For this review, use the dimensioned drawing (mm, ordinates from the lowest corner) and the shaded views. Give positions to 0.01 mm unless a question says otherwise; leave off trailing zeros. Loops run counter-clockwise (first coordinate to the right, second up) from the corner with the lowest first, then second, coordinate; pieces in that order, holes last. Notation, with made-up numbers: M 65.5,53.25 L 99.5,53.25 A11 cw 99.5,60.25 Z; hole C 10,14 d1. An arc over 180 degrees is marked long. Return JSON: item names as keys, results as strings.
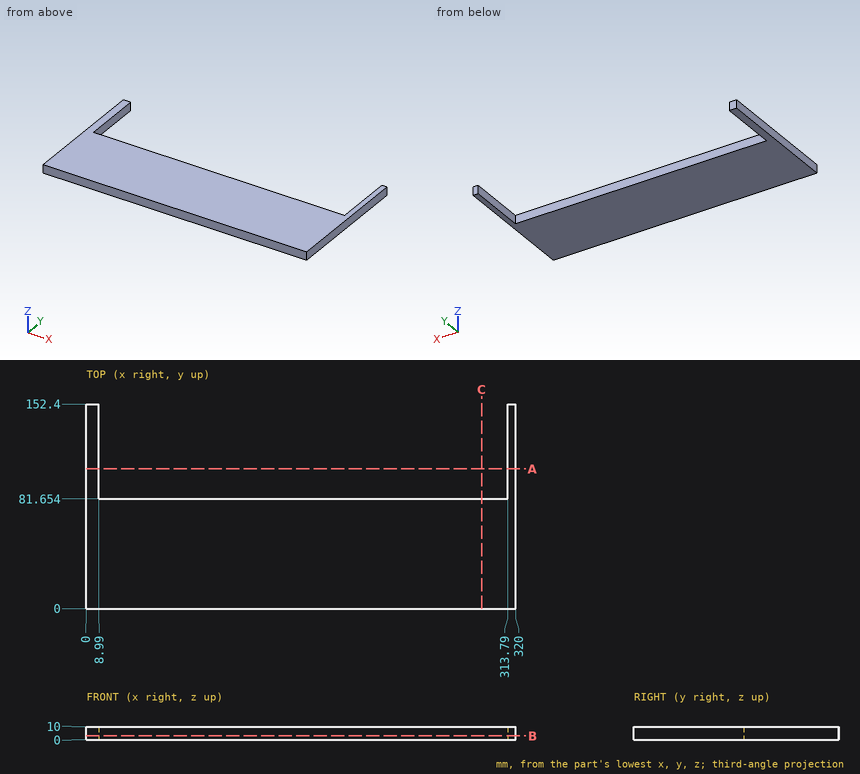
1) Insertion check: pin 1 (1 mm diameter, centred on x = 122.5, z = 5, fed in from +Y). The pin has a flat end and moves straight along its axis. Give the tip position at first contact, or say it passes through.
From the geometry:
{"pin 1": "y = 81.65"}
2) Consider section B-B on z = 3. Write out the cut boundary in (x, y), then the cut area to 3 significant figures.
From the geometry:
{"outline": "M 0,0 L 320,0 L 320,152.4 L 313.79,152.4 L 313.79,81.65 L 8.99,81.65 L 8.99,152.4 L 0,152.4 Z", "area": "27,200 mm²"}
3) Wall thickness on L1, parallel to X at y = 91, z = 5.5; L2, parallel to Y at x = 282, z = 6.75: over which ranges is each line inside the solid? List them lowest first. Write a range as from..to.
From the geometry:
{"L1": "0..8.99, 313.79..320", "L2": "0..81.65"}
4) Consider section A-A on y = 104. Write out the cut boundary in (x, z), then the cut area to 3 significant figures.
From the geometry:
{"outline": "M 0,0 L 8.99,0 L 8.99,10 L 0,10 Z; M 313.79,0 L 320,0 L 320,10 L 313.79,10 Z", "area": "152 mm²"}
5) Consider section C-C on x = 294.5. Write out the cut boundary in (y, z).
From the geometry:
{"outline": "M 0,0 L 81.65,0 L 81.65,10 L 0,10 Z"}
